```python
from build123d import *

# Parameters (mm, degrees)
F0_R      = 35
F1_DEPTH  = 50
F3_D      = 8
F3_DEPTH  = 10
F3_TIP    = 2.4034424761
F6_DEPTH  = 5
F9_DEPTH  = 5
F11_D     = 8.8
F11_DEPTH = 22.7505
F11_TIP   = 2.6437867237
F12_R     = 0.5


with BuildPart() as f1:
    # F0 (on Front) → F1 (new body)
    with BuildSketch(Plane.XZ):
        Circle(F0_R)
    extrude(amount=F1_DEPTH)

    # F3
    with Locations(Plane.XZ.offset(50)):
        with Locations((0, 28), (0, 0), (20, -10), (-20, -10)):
            Hole(F3_D / 2, depth=F3_DEPTH)
            with Locations((0, 0, -(F3_DEPTH + F3_TIP / 2))):  # 118° drill point
                Cone(0, F3_D / 2, F3_TIP, mode=Mode.SUBTRACT)

    # F5 (on offset) → F6 (cut)
    with BuildSketch(Plane.YZ.offset(35)):
        with BuildLine():
            Line((-10.0009293836, 3.999999892), (-39.764888731, 3.9930843581))
            ThreePointArc((-39.764888731, 3.9930843581), (-43.9989519, 0.0915625537), (-39.947895719, -3.9996606286))
            Line((-39.947895719, -3.9996606286), (-10.0000453283, -3.9999999997))
            ThreePointArc((-10.0000453283, -3.9999999997), (-6.0000000244, 0.0004420276), (-10.0009293836, 3.999999892))
        make_face()
    extrude(amount=-F6_DEPTH, mode=Mode.SUBTRACT)

    # F8 (on offset) → F9 (cut)
    with BuildSketch(Plane.YZ.offset(-35)):
        with BuildLine():
            Line((-10.0013998348, 3.775364694), (-39.764888731, 3.7649502201))
            ThreePointArc((-39.764888731, 3.7649502201), (-43.9989519, -0.1365715843), (-39.947895719, -4.2277947666))
            Line((-39.947895719, -4.2277947666), (-9.99957818, -4.2246350388))
            ThreePointArc((-9.99957818, -4.2246350388), (-6.0000003078, -0.2237242337), (-10.0013998348, 3.775364694))
        make_face()
    extrude(amount=F9_DEPTH, mode=Mode.SUBTRACT)

    # F11
    with Locations(Plane(origin=(0, 0, 0), x_dir=(1, 0, 0), z_dir=(0, 1, 0))):
        with Locations((0, 0)):
            Hole(F11_D / 2, depth=F11_DEPTH)
            with Locations((0, 0, -(F11_DEPTH + F11_TIP / 2))):  # 118° drill point
                Cone(0, F11_D / 2, F11_TIP, mode=Mode.SUBTRACT)

    # F12
    f12_edges = [f1.edges().sort_by_distance(p)[0] for p in [
        (-35, -50, 0),
        (-35, 0, 0),
    ]]
    fillet(f12_edges, radius=F12_R)


solid = f1.part
```
Read the model definition and answer for the solid it produces. Units are mm, in the model's axes. A direction names the side the tool comes from. Round coordinates to 2 decimals unless told otherwise and drop trailing zeros. Write each loop counter-clockwise with the first axis right and the second up, starting at its lowest first coordinate (ties: lowest second). Pieces come first, ordered by that corner, then holes. Notation, with made-up numbers: (35, -6.75) - (54, -6.75) arc R11 cw to (54, 10.25) - close; hole circle Ø3 at (-12, -31.75). An arc over 180 degrees is marked (long way). One line per item, written item: value.
Q1. Which of the six approach directions +Z, -Z, +X, -X, +Y, -Y give full straight-line access (tool end or side, diameter ignored) to faces 4 (the flat face through (30, -25, 0)), 5 (the cylindrical face through (-4.197, -11.535, -1.322)), 6 (the cylindrical face through (0.867, -44.93, -3.905)), 7 (the cylindrical face through (-32.5, -6, -0.3))?
The answers:
face 4: +X
face 5: +Y
face 6: -Y
face 7: -X
Q2. Straight lines are drawn through the part: line 1 (X direction, y = -43, z = 0); line 2 (X direction, y = -46.5, z = -13); line 3 (X direction, y = -46.75, z = -10). For each, find the intervals that lie inside material, in ascending order. Write a range as from..to.
The answers:
line 1: x = -30..-4, 4..30
line 2: x = -32.5..-22.65, -17.35..17.35, 22.65..32.5
line 3: x = -33.54..-24, -16..16, 24..33.54
Q3. Each of these flat-tipped pins is pushed along its axis until it touches: P1, Ø8, axis at y = -20.5, z = 22, coming from the +X side; P2, Ø6.5, axis at x = 0, z = 0, coming from the +Y side; P3, Ø9, axis at y = -23, z = -1.5, coming from the -X side. Where does it stop, or does it pass through?
The answers:
P1: stops at x = 30.02
P2: stops at y = -23.44
P3: stops at x = -34.74
Q4. For a pull along Z with two mould halves and no side action, classify faces 1 (the cylindrical face through (23.2, -44.9, -12.4)), 2 (the cylindrical face through (32.33, -24.66, -13.41)), 3 (the flat face through (0, -50, -7)) as pulls with the +Z half, pulls with the -Z half, needs draft (parallel to the pull), parting line crosses it, or undercut.
The answers:
face 1: undercut
face 2: parting line crosses it
face 3: needs draft
Q5. Find section A-A (y = -11.5). Determine the outline of the cut face in (x, z).
The answers:
outline: (-34.8, 3.77) - (-30, 3.77) - (-30, -4.22) - (-34.74, -4.22) arc R35 ccw to (34.77, -4) - (30, -4) - (30, 4) - (34.77, 4) arc R35 ccw to start; hole circle Ø8.8 at (0, 0)
Q6. Find section C-C (y = -3.5). Determine the outline of the cut face in (x, z), and give its area (3 significant figures).
The answers:
outline: circle Ø70 at (0, 0); hole circle Ø8.8 at (0, 0)
area: 3,790 mm2
Q7. Find section B-B (y = -18). Determine the outline of the cut face in (x, z), and give its area (3 significant figures).
The answers:
outline: (-34.8, 3.77) - (-30, 3.77) - (-30, -4.23) - (-34.74, -4.23) arc R35 ccw to (34.77, -4) - (30, -4) - (30, 4) - (34.77, 4) arc R35 ccw to start; hole circle Ø8.8 at (0, 0)
area: 3,710 mm2
